Check sheet for the drawn part. Datum: minimum x, y, z corner. Units: mm. A direction names the side the tool comes from. Give positions to 0.01 mm unless a question says otherwise; leave off trailing zeros. Write each loop counter-clockwise with the first axis right and the second up, starting at its lowest first coordinate (ties: lowest second). Pieces come first, ordered by that corner, then holes.
(1) Depth check by flat-ended pin: P1, Ø6.5, axis at y = 97.5, z = 80, coming from the -X side; P2, Ø6, axis at x = 49.5, z = 156, coming from the +Y side. Enter the tip coordinate at first touch or a pass-through.
(2) Cross-section at A-A (z = 80). Count the separate pieces of the cut face and the enclosed holes in it, and give its area (3 significant figures).
(3) Cross-section at C-C (z = 50). Record the boundary of the cut face in (x, y), and give its area (3 significant figures).
(4) Tool access check on the marked faces 1 and 2. Record the directions out of +Z, -Z, +X, -X, +Y, -Y that give a thin tool (end or side, any length) a straight path to the whole face; none if there is none.
(5) Cross-section at D-D (y = 10). Record the boundary of the cut face in (x, z).
(6) Mould release check, pull along X, two halves, no side actions. Record for the marked faces 3, 4 and 5: +X half, -X half, draft (parallel to the pull), parting line (faces both ways), or undercut.
(7) Thickness scan on line 1 along Z through (x, y) = (363, 97.5); line 2 along Y through (x, z) = (361, 80); line 3 along X through (y, z) = (62, 193). Record the ranges inside material, lowest first.
(8) Cross-section at B-B (y = 108). Record the boundary of the cut face in (x, z).
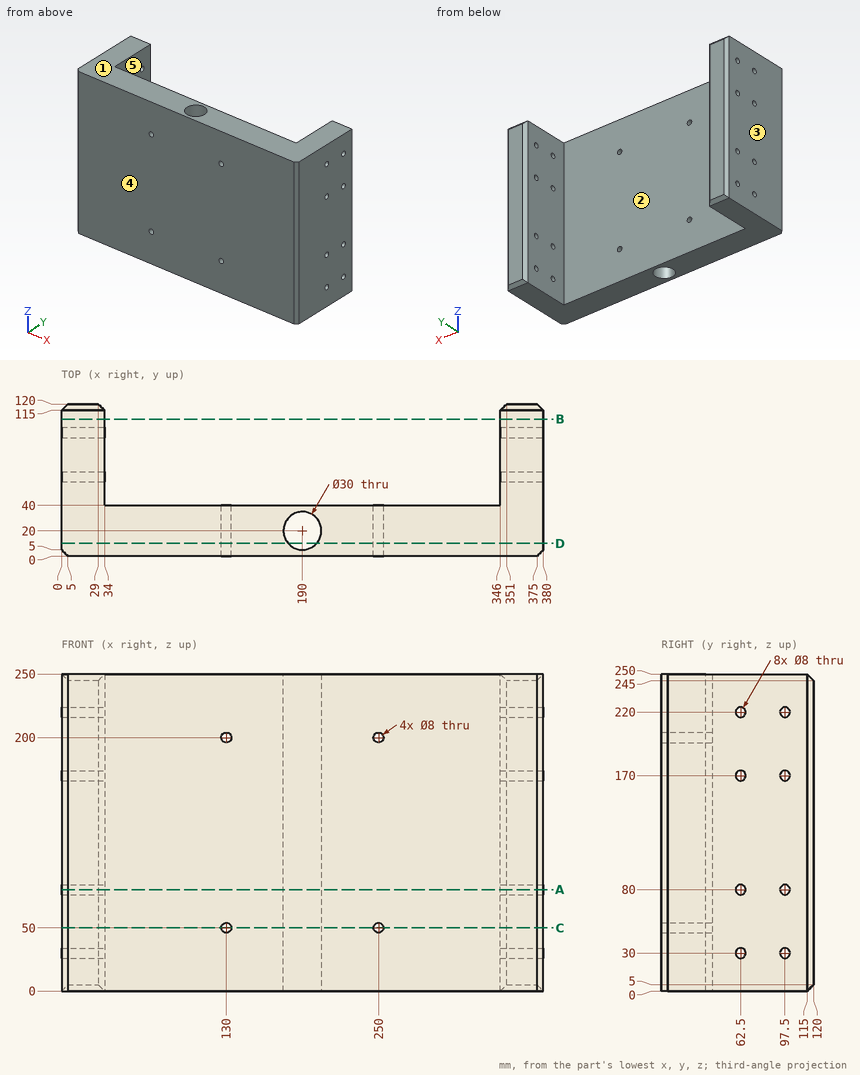
Reply:
1. P1: passes through
1. P2: stops at y = 40
2. separate pieces: 5
2. enclosed holes: 1
2. area: 18,800 mm2
3. outline: (0, 5) - (5, 0) - (126, 0) - (126, 40) - (34, 40) - (34, 115) - (29, 120) - (5, 120) - (0, 115) - close; (134, 0) - (246, 0) - (246, 40) - (134, 40) - close; (254, 0) - (375, 0) - (380, 5) - (380, 115) - (375, 120) - (351, 120) - (346, 115) - (346, 40) - (254, 40) - close; hole circle Ø30 at (190, 20)
3. area: 19,200 mm2
4. face 1: +Z, +X, -X, +Y, -Y
4. face 2: +Z, -Z, +Y
5. outline: (0, 0) - (178.82, 0) - (178.82, 250) - (0, 250) - close; (201.18, 0) - (380, 0) - (380, 250) - (201.18, 250) - close; hole circle Ø8 at (130, 50); hole circle Ø8 at (130, 200); hole circle Ø8 at (250, 50); hole circle Ø8 at (250, 200)
6. face 3: -X half
6. face 4: draft
6. face 5: undercut
7. line 1: z = 0 to 26, 34 to 76, 84 to 166, 174 to 216, 224 to 250
7. line 2: y = 0 to 58.5, 66.5 to 93.5, 101.5 to 120
7. line 3: x = 0 to 34, 346 to 380
8. outline: (0, 0) - (34, 0) - (34, 250) - (0, 250) - close; (346, 0) - (380, 0) - (380, 250) - (346, 250) - close
